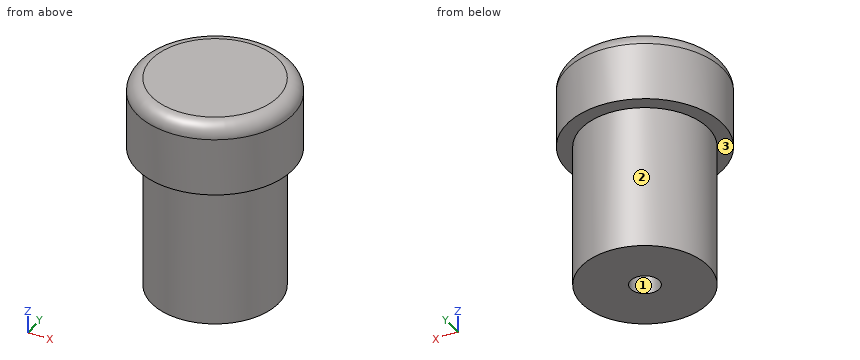
```python
from build123d import *

# Parameters (mm, degrees)
SKETCH_1_R          = 10.8
EXTRUDE_1_DEPTH     = 10
SKETCH_2_R          = 8.8
EXTRUDE_2_DEPTH     = 20
FILLET_1_R          = 2
SKETCH_3_R          = 2
CUT_EXTRUDE_1_DEPTH = 10


with BuildPart() as part:
    # 草图1 → 凸台-拉伸1 (new body)
    with BuildSketch(Plane.XY):
        Circle(SKETCH_1_R)
    extrude(amount=EXTRUDE_1_DEPTH)

    # 草图2 → 凸台-拉伸2 (add)
    with BuildSketch(Plane(origin=(0, 0, 0), x_dir=(-1, 0, 0), z_dir=(0, 0, -1))):
        Circle(SKETCH_2_R)
    extrude(amount=EXTRUDE_2_DEPTH)

    # 圆角1
    fillet_1_edges = [part.edges().sort_by_distance(p)[0] for p in [
        (-10.8, 0, 10),
    ]]
    fillet(fillet_1_edges, radius=FILLET_1_R)

    # 草图3 → 切除-拉伸1 (cut)
    with BuildSketch(Plane(origin=(0, 0, -20), x_dir=(-1, 0, 0), z_dir=(0, 0, -1))):
        Circle(SKETCH_3_R)
    extrude(amount=-CUT_EXTRUDE_1_DEPTH, mode=Mode.SUBTRACT)


solid = part.part
```
Read the model definition and answer for the solid it produces. Units are mm, in the model's axes. Face numbers are marked on the shaded views. Coordinates: 2 decimals unless noted, no trailing zeros. Order: outer loops, then holes, each group sorted by start corner. A loop starts at its lowest first (then second) coordinate and runs counter-clockwise, first axis right, second up. Notation, with made-up numbers: (25.5, -12) - (30.5, -12) arc R12 ccw to (30.5, 9) - close; hole circle Ø5 at (43.5, 56.5). An arc over 180 degrees is marked (long way). Answer as a JSON object with one key per item and string values. Group by question number.
Item 1: The mould has two halves that part along X. Classify the marked faces 1, 2 and 3: +X half, -X half, draft (parallel to the pull), parting line (faces both ways), or undercut.
Item 2: Section D-D (z = 7) is taken. Give the vertices of the cut face in (x, y).
Item 3: Section A-A (y = 0) is taken. Give the vertices of the cut face in (x, z).
Item 4: Flat-ended cylindrical pins translate along their axes: P1, Ø4, axis at y = -5.5, z = -1.5, coming from the +X side; P2, Ø3.5, axis at x = 0, y = 0, coming from the -Z side; P3, Ø5, axis at x = -8.5, z = -15, coming from the -Y side. Find the tip coordinate at first contact, or state that the pin passes through.
Item 5: Consider probe 1 along Y at (x, z) = (0, -13.75); probe 2 along X at (y, z) = (-7.75, 1.75); probe 3 along Y at (x, z) = (-1.25, -17.5). Determine where each line is inside the solid, lowest interval first. Write a range as from..to.
Item 6: Section C-C (z = -16) is taken. Give the vertices of the cut face in (x, y).
Results are:
{
 "1": {"face 1": "undercut", "face 2": "parting line", "face 3": "draft"},
 "2": {"outline": "circle Ø21.6 at (0, 0)"},
 "3": {"outline": "(-10.8, 0) - (-8.8, 0) - (-8.8, -20) - (-2, -20) - (-2, -10) - (2, -10) - (2, -20) - (8.8, -20) - (8.8, 0) - (10.8, 0) - (10.8, 8) arc R2 ccw to (8.8, 10) - (-8.8, 10) arc R2 ccw to (-10.8, 8) - close"},
 "4": {"P1": "stops at x = 9.96", "P2": "stops at z = -10", "P3": "stops at y = -6.44"},
 "5": {"probe 1": "y = -8.8..-2, 2..8.8", "probe 2": "x = -7.52..7.52", "probe 3": "y = -8.71..-1.56, 1.56..8.71"},
 "6": {"outline": "circle Ø17.6 at (0, 0); hole circle Ø4 at (0, 0)"}
}
